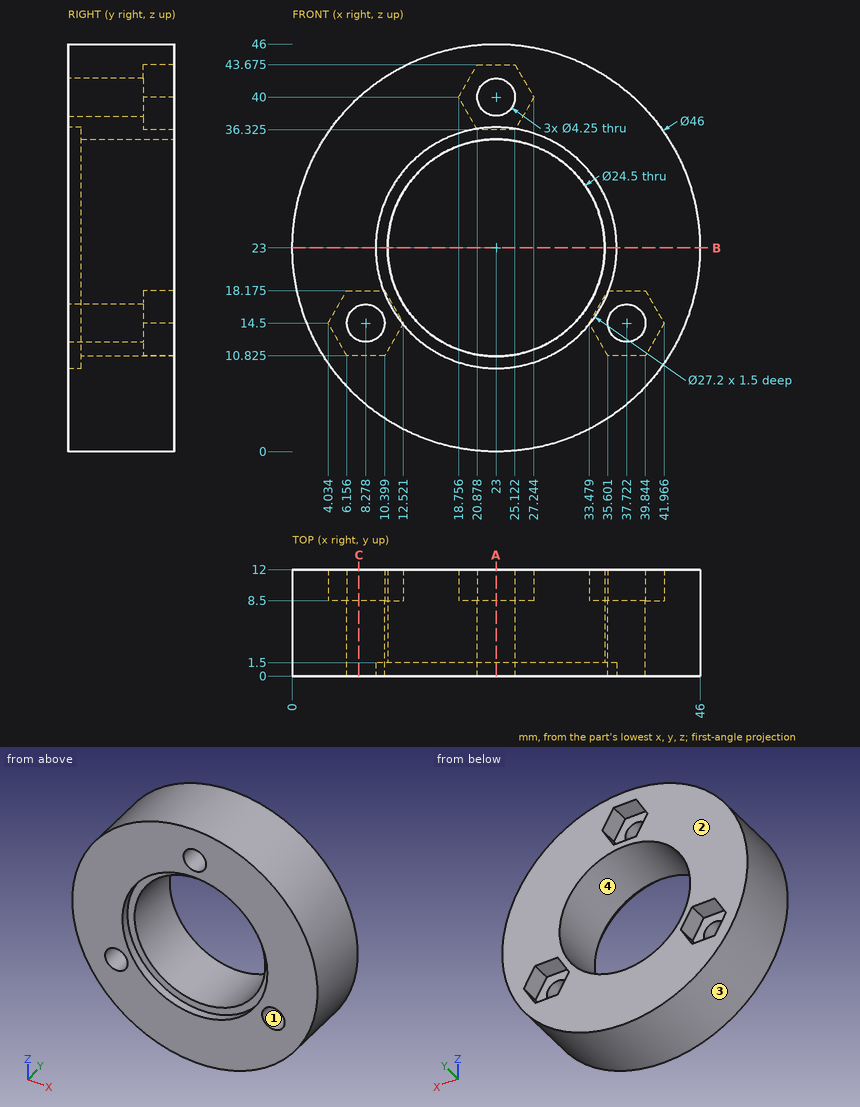
Geometry: see drawing. Coordinates: mm, zero at the bounding-box minimum. Round coordinates to 2 decimals unless told otherwise and drop trailing zeros. Loops run counter-clockwise (first coordinate to the right, second up) from the corner with the lowest first, then second, coordinate; pieces in that order, holes last. Notation, with made-up numbers: M 6,-26.5 L 21,-26.5 A26 cw 21,-5.5 Z; hole C 58.5,56 d5. An arc over 180 degrees is marked long. Use a Markdown table: item, result. Add a question column.
1. Section query A-A on x = 23. Give the number of separate pieces and of enclosed holes in the cut face, then the cut area to 3 significant figures.
2. Line query: line 1 (Z direction, x = 36, y = 9) (1 decimal); line 2 (X direction, y = 4.25, z = 23.5) (1 decimal); line 3 (Y direction, x = 34.5, z = 14.5). Output: solid intervals per line, ascending.
3. Mould query, pull axis X, two halves, no side actions, for the marked faces 1, 2, 3 and 4. Classes: pulls with the +X half, pulls with the -X half, needs draft (parallel to the pull), parting line crosses it, or undercut.
4. Section query C-C on x = 7.5. Return the cut outline in (y, z) (1 decimal).
5. Section query B-B on z = 23. Return the cut outline in (x, y), then the cut area to 3 significant figures.
6. Contact query for flat-ended pins moving along their axis: P1, Ø6, axis at x = 12, z = 18, coming from the -Y side; P2, Ø1, axis at x = 37, y = 10.5, coming from the +Z side; P3, Ø4, axis at x = 37.72, z = 14.5, coming from the +Y side; P4, Ø4, axis at x = 13.5, y = 3.5, coming from the -Z side. Output: stop coordinate, or through.
Reported:
| question | item | result |
|---|---|---|
| 1 | separate pieces | 3 |
| 1 | enclosed holes | 0 |
| 1 | area | 192 mm² |
| 2 | line 1 | z = 4 to 10.8, 18.2 to 42 |
| 2 | line 2 | x = 0 to 10.8, 35.2 to 46 |
| 2 | line 3 | y = 0 to 8.5 |
| 3 | face 1 | undercut |
| 3 | face 2 | needs draft |
| 3 | face 3 | parting line crosses it |
| 3 | face 4 | undercut |
| 4 | outline | M 0,6 L 12,6 L 12,10.8 L 8.5,10.8 L 8.5,12.5 L 0,12.5 Z; M 0,16.5 L 8.5,16.5 L 8.5,18.2 L 12,18.2 L 12,40 L 0,40 Z |
| 5 | outline | M 0,0 L 9.4,0 L 9.4,1.5 L 10.75,1.5 L 10.75,12 L 0,12 Z; M 35.25,1.5 L 36.6,1.5 L 36.6,0 L 46,0 L 46,12 L 35.25,12 Z |
| 5 | area | 254 mm² |
| 6 | P1 | stops at y = 0 |
| 6 | P2 | stops at z = 41.62 |
| 6 | P3 | passes through |
| 6 | P4 | stops at z = 1.26 |
